The model under review builds one solid part; all positions refer to its coordinate system, in mm. A direction names the side the tool comes from. Coordinates: 2 decimals unless noted, no trailing zeros. Order: outer loops, then holes, each group sorted by start corner. A loop starts at its lowest first (then second) coordinate and runs counter-clockwise, first axis right, second up.
Autodesk Inventor part; units mm, degrees
ref_plane "YZ Plane" through (0, 0, 0) normal (1, 0, 0) x (0, 1, 0)
ref_plane "XZ Plane" through (0, 0, 0) normal (0, 1, 0) x (-1, 0, 0)
ref_plane "XY Plane" through (0, 0, 0) normal (0, 0, 1) x (1, 0, 0)
sketch "Náčrt1" plane through (0, 0, 0) normal (0, 0, 1) x (1, 0, 0)
  line L0 (-4, 1.45) -> (4, 1.45)
  line L1 (4, 1.45) -> (4, -1.45)
  line L2 (4, -1.45) -> (-4, -1.45)
  line L3 (-4, -1.45) -> (-4, 1.45)
  line L4 (-4, 1.45) -> (4, -1.45) construction
  line L5 (4, 1.45) -> (-4, -1.45) construction
  line L6 (-3, 1) -> (3, 1)
  line L7 (3, 1) -> (3, -1)
  line L8 (3, -1) -> (-3, -1)
  line L9 (-3, -1) -> (-3, 1)
  line L10 (-3, 1) -> (3, -1) construction
  line L11 (3, 1) -> (-3, -1) construction
  line L12 (-3, 0.67) -> (-3.5, 0.67)
  line L13 (-3.5, 0.67) -> (-3.5, 0.05)
  line L14 (-3.5, 0.05) -> (-3, 0.05)
  line L15 (3, 0.67) -> (3.5, 0.67)
  line L16 (3.5, 0.67) -> (3.5, 0.05)
  line L17 (3.5, 0.05) -> (3, 0.05)
  point P0 (0, 0)
  dimension "d0" = 8
  dimension "d1" = 2.9
  dimension "d2" = 2
  dimension "d3" = 6
  dimension "d4" = 7
  dimension "d5" = 0.62
  dimension "d6" = 1.5
extrude "Vysunutí1" add sketch "Náčrt1" along normal blind 4.25
extrude "Vysunutí2" add sketch "Náčrt1" along normal blind 1.25 contours L6 L7 L8 L9 | L9 L14 L13 L12 | L15 L16 L17 L7
sketch "Náčrt2" plane through (0, 0, 1.25) normal (0, 0, 1) x (1, 0, 0)
  line L0 (-2.65, 0.67) -> (-2.35, 0.67)
  line L1 (-2.35, 0.67) -> (-2.35, 0.37)
  line L2 (-2.35, 0.37) -> (-2.65, 0.37)
  line L3 (-2.65, 0.37) -> (-2.65, 0.67)
  line L4 (-2.65, 0.67) -> (-2.35, 0.37) construction
  line L5 (-2.35, 0.67) -> (-2.65, 0.37) construction
  line L6 (-1.65, 0.67) -> (-1.35, 0.67)
  line L7 (-1.35, 0.67) -> (-1.35, 0.37)
  line L8 (-1.35, 0.37) -> (-1.65, 0.37)
  line L9 (-1.65, 0.37) -> (-1.65, 0.67)
  line L10 (-1.65, 0.67) -> (-1.35, 0.37) construction
  line L11 (-1.35, 0.67) -> (-1.65, 0.37) construction
  line L12 (-0.65, 0.67) -> (-0.35, 0.67)
  line L13 (-0.35, 0.67) -> (-0.35, 0.37)
  line L14 (-0.35, 0.37) -> (-0.65, 0.37)
  line L15 (-0.65, 0.37) -> (-0.65, 0.67)
  line L16 (-0.65, 0.67) -> (-0.35, 0.37) construction
  line L17 (-0.35, 0.67) -> (-0.65, 0.37) construction
  line L18 (0.35, 0.67) -> (0.65, 0.67)
  line L19 (0.65, 0.67) -> (0.65, 0.37)
  line L20 (0.65, 0.37) -> (0.35, 0.37)
  line L21 (0.35, 0.37) -> (0.35, 0.67)
  line L22 (0.35, 0.67) -> (0.65, 0.37) construction
  line L23 (0.65, 0.67) -> (0.35, 0.37) construction
  line L24 (1.35, 0.67) -> (1.65, 0.67)
  line L25 (1.65, 0.67) -> (1.65, 0.37)
  line L26 (1.65, 0.37) -> (1.35, 0.37)
  line L27 (1.35, 0.37) -> (1.35, 0.67)
  line L28 (1.35, 0.67) -> (1.65, 0.37) construction
  line L29 (1.65, 0.67) -> (1.35, 0.37) construction
  line L30 (2.35, 0.67) -> (2.65, 0.67)
  line L31 (2.65, 0.67) -> (2.65, 0.37)
  line L32 (2.65, 0.37) -> (2.35, 0.37)
  line L33 (2.35, 0.37) -> (2.35, 0.67)
  line L34 (2.35, 0.67) -> (2.65, 0.37) construction
  line L35 (2.65, 0.67) -> (2.35, 0.37) construction
  line L36 (-3, -1) -> (-3, 0.05)
  line L37 (-3, 0.37) -> (-2.65, 0.37) construction
  line L38 (2.65, 0.37) -> (3, 0.37) construction
  line L39 (3, 0.05) -> (3, -1) construction
  point P0 (0, 0)
  point P1 (-2.5, 0.52)
  point P2 (-1.5, 0.52)
  point P3 (-0.5, 0.52)
  point P4 (0.5, 0.52)
  point P5 (1.5, 0.52)
  point P6 (2.5, 0.52)
  point P7 (-3, 0.67)
  dimension "d13" = 1
  dimension "d19" = 0.3
  dimension "d20" = 0.3
extrude "Vysunutí3" add sketch "Náčrt2" along normal blind 2
properties part number "jst - 1 mm 6 pin female"
(1) We need section C-C, the plane x = -0.5. Write out the cut boundary in (y, z).
A:
outline: (-1.45, 0) - (1.45, 0) - (1.45, 4.25) - (1, 4.25) - (1, 1.25) - (0.67, 1.25) - (0.67, 3.25) - (0.37, 3.25) - (0.37, 1.25) - (-1, 1.25) - (-1, 4.25) - (-1.45, 4.25) - close
(2) We need section A-A, the plane z = 3.45. Write out the cut boundary in (x, y).
A:
outline: (-4, -1.45) - (4, -1.45) - (4, 1.45) - (-4, 1.45) - close; hole (-3.5, 0.05) - (-3, 0.05) - (-3, -1) - (3, -1) - (3, 0.05) - (3.5, 0.05) - (3.5, 0.67) - (3, 0.67) - (3, 1) - (-3, 1) - (-3, 0.67) - (-3.5, 0.67) - close
(3) We need section D-D, the plane z = 2.25. Count the separate pieces of the cut face and the enclosed holes in it, and give its area (3 significant figures).
A:
separate pieces: 7
enclosed holes: 1
area: 11.1 mm2
(4) We need section B-B, the plane y = -0.1. Write out the cut boundary in (x, z).
A:
outline: (-4, 0) - (4, 0) - (4, 4.25) - (3, 4.25) - (3, 1.25) - (-3, 1.25) - (-3, 4.25) - (-4, 4.25) - close
(5) For pin 1 Ø1 at (x, y) = (3, 0.5) entering from -Z, flat-tipped, find the tip position at first contact; note if it passes through.
A:
pin 1: stops at z = 0
(6) Draft analysis for pull direction Y (two halves, no side actions). For faces 1 (the face through (0, -1.45, 2)), 2 (the face through (0, 1, 3)), 3 (the face through (-0.06, -1.27, 4.25)), state which applies: released by +Y, released by -Y, zero draft, split by the parting line, or undercut.
A:
face 1: released by -Y
face 2: undercut
face 3: zero draft
(7) Wall thickness on probe 1 along Y at (x, z) = (-2.5, 2.2); probe 2 along Y at (x, z) = (1, 3.65); probe 3 along X at (y, z) = (-0.35, 3.75): over which ranges is each line inside the solid? List them lowest first.
A:
probe 1: y = -1.45 to -1, 0.37 to 0.67, 1 to 1.45
probe 2: y = -1.45 to -1, 1 to 1.45
probe 3: x = -4 to -3, 3 to 4
(8) Machinability: for faces 4 (the face through (4, 0, 2)), 5 (the face through (0, -1, 3)), which of the approach directions +Z, -Z, +X, -X, +Y, -Y give a long, thin tool a straight path to every point of the face, cutting with its end or side? Answer none if there is none.
A:
face 4: +Z, -Z, +X, +Y, -Y
face 5: +Z
